Autodesk Inventor part; units mm, degrees
ref_plane "YZ Plane" through (0, 0, 0) normal (1, 0, 0) x (0, 1, 0)
ref_plane "XZ Plane" through (0, 0, 0) normal (0, 1, 0) x (-1, 0, 0)
ref_plane "XY Plane" through (0, 0, 0) normal (0, 0, 1) x (1, 0, 0)
sketch "Sketch1" plane through (0, 0, 0) normal (0, 0, 1) x (1, 0, 0)
  circle A0 centre (0, 0) radius 4.55
  dimension "d0" = 9.1
extrude "Base" add sketch "Sketch1" along normal blind 0.71
sketch "Sketch2" plane through (0, 0, 0.71) normal (0, 0, 1) x (1, 0, 0)
  circle A0 centre (0, 0) radius 4.15
  dimension "d3" = 8.3
extrude "Can: Outer Wall" add sketch "Sketch2" along normal blind 3.9
sketch "Sketch3" plane through (0, 0, 4.61) normal (0, 0, 1) x (1, 0, 0)
  circle A0 centre (0, 0) radius 3.85
  dimension "d6" = 7.7
extrude "Can: Inner Wall" cut sketch "Sketch3" against normal blind 3.9
sketch "Sketch4" plane through (0, 0, 4.61) normal (0, 0, 1) x (1, 0, 0)
  circle A0 centre (0, 0) radius 3.85
  dimension "d9" = 7.7
extrude "Can: Top" add sketch "Sketch4" against normal blind 0.3
sketch "Sketch5" plane through (0, 0, 4.61) normal (0, 0, 1) x (1, 0, 0)
  circle A0 centre (0, 0) radius 3.05
  dimension "d12" = 6.1
extrude "Can: Hole" cut sketch "Sketch5" against normal blind 0.3
ref_plane "Work Plane1" through (0, 0, 4.31) normal (0, 0, 1) x (1, 0, 0)
sketch "Sketch8" plane through (0, 0, 4.31) normal (0, 0, 1) x (1, 0, 0)
  circle A0 centre (0, 0) radius 3.15
  dimension "d16" = 6.3
extrude "Window" add sketch "Sketch8" against normal blind 0.1
sketch "Sketch9" plane through (0, 0, 0) normal (0, 0, -1) x (-1, 0, 0)
  line L0 (0, -0.4) -> (-5.15, -0.4)
  line L1 (-5.15, -0.4) -> (-5.15, 0.4)
  line L2 (-5.15, 0.4) -> (0, 0.4)
  line L3 (0, 0.4) -> (0, -0.4)
  point P0 (0, 0)
  dimension "d19" = 5.15
  dimension "d20" = 0.8
extrude "Key" add sketch "Sketch9" against normal blind 0.7
sketch "Sketch10" plane through (0, 0, 0) normal (0, 0, -1) x (-1, 0, 0)
  circle A0 centre (-1.803, 1.803) radius 0.25
  point P0 (0, 0)
  dimension "d23" = 0.5
extrude "Pin 1" add sketch "Sketch10" along normal blind 38
sketch "Sketch11" plane through (0, 0, 0) normal (0, 0, -1) x (-1, 0, 0)
  circle A0 centre (1.803, 1.803) radius 0.25
  point P0 (0, 0)
  dimension "d26" = 0.5
extrude "Pin 2" add sketch "Sketch11" along normal blind 38
sketch "Sketch12" plane through (0, 0, 0) normal (0, 0, -1) x (-1, 0, 0)
  circle A0 centre (1.803, -1.803) radius 0.25
  point P0 (0, 0)
  dimension "d29" = 0.5
extrude "Pin 3" add sketch "Sketch12" along normal blind 38
properties part number "Thorlabs_FDS010" material "Gold"
The listing builds one solid part. Answer for the finished solid, in the listing's coordinates (mm). Coordinates: 2 decimals unless noted, no trailing zeros. Order: outer loops, then holes, each group sorted by start corner. A loop starts at its lowest first (then second) coordinate and runs counter-clockwise, first axis right, second up. Notation, with made-up numbers: (78, 82) -> (110, 82) arc R20 ccw to (110, 98) -> close; hole circle Ø5 at (4.5, 19). An arc over 180 degrees is marked (long way). Answer in a Markdown table with one row per item. Add a question column.
Item 1: Find section C-C (z = -26). Write down the section's boundary in (x, y), then the cut area to 3 significant figures.
Item 2: Find section B-B (x = 0). Write down the section's boundary in (y, z).
Item 3: Each of these flat-tipped pins is pushed along its axis until it touches: P1, Ø0.7, axis at x = 5, z = 0, coming from the +Y side; P2, Ø0.7, axis at x = 5, y = 0, coming from the +Z side; P3, Ø2.5, axis at x = 1.5, y = 0, coming from the -Z side. Where does it stop, or does it pass through?
Item 4: Determine the mould class of faces 1 (the face through (2.91, 0.92, 4.46)), 2 (the face through (-0.9, 4.05, 2.63)), 3 (the face through (-2, 3, 4.61)) for opening direction X: +X half, -X half, draft (parallel to the pull), parting line (faces both ways), or undercut.
Item 5: Find the intervals of material crossed by L1, parallel to Y at x = 0, z = 3.05; L2, parallel to Y at x = 0, z = 4.55; L3, parallel to Z at x = -2.5, y = 3.5, in increasing order. Write a range as from..to.
Result set:
| question | item | result |
|---|---|---|
| 1 | outline | circle Ø0.5 at (-1.8, -1.8); circle Ø0.5 at (-1.8, 1.8); circle Ø0.5 at (1.8, 1.8) |
| 1 | area | 0.589 mm² |
| 2 | outline | (-4.55, 0) -> (4.55, 0) -> (4.55, 0.71) -> (4.15, 0.71) -> (4.15, 4.61) -> (3.05, 4.61) -> (3.05, 4.31) -> (-3.05, 4.31) -> (-3.05, 4.61) -> (-4.15, 4.61) -> (-4.15, 0.71) -> (-4.55, 0.71) -> close; hole (-3.85, 0.71) -> (3.85, 0.71) -> (3.85, 4.31) -> (3.15, 4.31) -> (3.15, 4.21) -> (-3.15, 4.21) -> (-3.15, 4.31) -> (-3.85, 4.31) -> close |
| 3 | P1 | stops at y = 0.4 |
| 3 | P2 | stops at z = 0.7 |
| 3 | P3 | stops at z = 0 |
| 4 | face 1 | undercut |
| 4 | face 2 | parting line |
| 4 | face 3 | draft |
| 5 | L1 | y = -4.15..-3.85, 3.85..4.15 |
| 5 | L2 | y = -4.15..-3.05, 3.05..4.15 |
| 5 | L3 | z = 0..0.71 |
